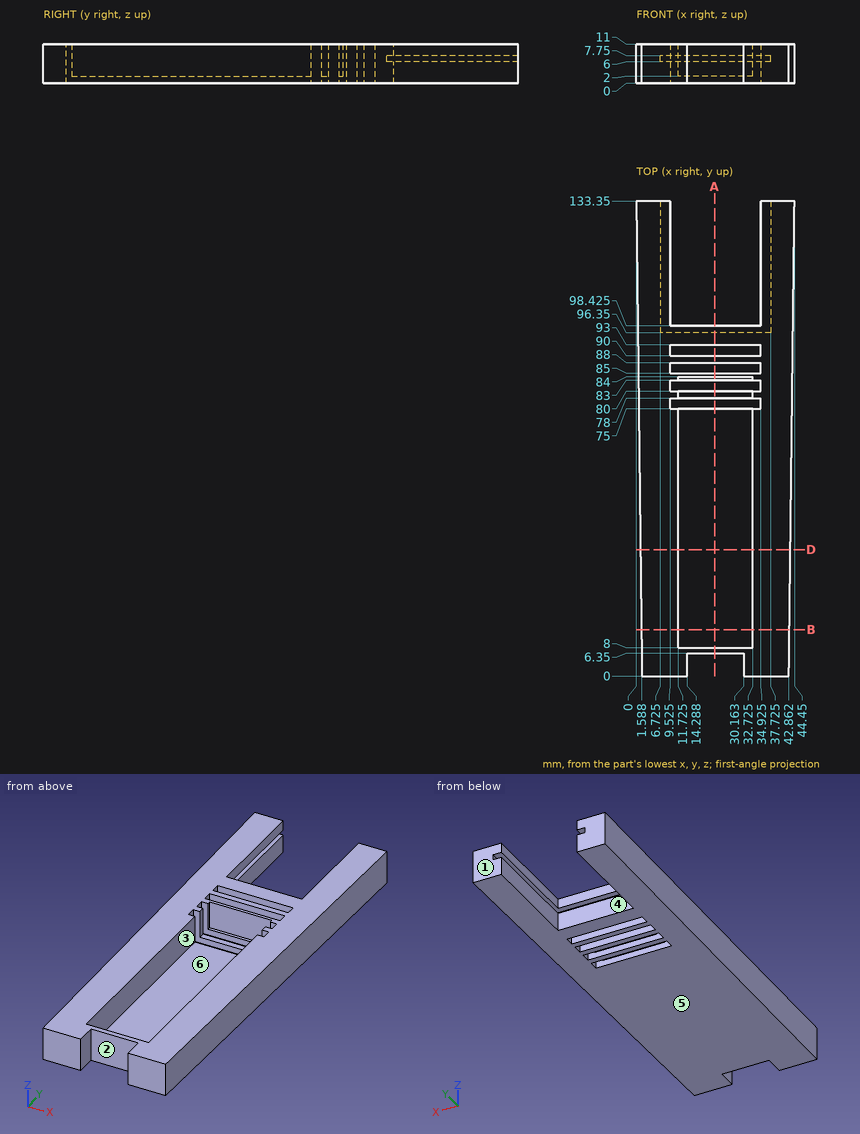
For this review, use the dimensioned drawing (mm, ordinates from the lowest corner) and the shaded views. A direction names the side the tool comes from. Give positions to 0.01 mm unless a question says otherwise; leave off trailing zeros. Order: outer loops, then holes, each group sorted by start corner. A loop starts at its lowest first (then second) coordinate and runs counter-clockwise, first axis right, second up.
1. Mouldability with a two-part tool opening along Y and no side actions: class the marked faces 1, 2 and 3 as +Y half, -Y half, draft (parallel to the pull), parting line (faces both ways), or undercut.
Solution:
face 1: +Y half
face 2: -Y half
face 3: undercut
2. For pin 1 Ø3.5 at (x, z) = (16.5, 3) entering from +Y (1 decimal); pin 2 Ø4 at (x, z) = (6.5, 3.5) entering from -Y; pin 3 Ø2 at (x, z) = (20, 2.5) entering from -Y; pin 4 Ø1 at (y, z) = (78.5, 7) entering from +X, all flat-tipped, find the tip position at first contact; note any pin that passes through.
Solution:
pin 1: stops at y = 98.4
pin 2: stops at y = 0
pin 3: stops at y = 6.35
pin 4: stops at x = 43.8
3. Tool access review of the marked faces 4, 5 and 6: name each direction out of +Z, -Z, +X, -X, +Y, -Y from which nothing blocks a thin tool from reaching the whole face with its end or side.
Solution:
face 4: +Z, -Z, +Y
face 5: -Z, +X, -X, +Y, -Y
face 6: +Z
4. To check wall thickness, follow L1, parallel to Y at x = 17, z = 7; L2, parallel to Y at x = 13, z = 4 (1 decimal); L3, parallel to Z at x = 19, y = 19. State the ranges of each line that lie inside material, in increasing order.
Solution:
L1: y = 6.35 to 8, 84 to 85, 88 to 90, 93 to 96.35
L2: y = 0 to 8, 84 to 85, 88 to 90, 93 to 98.4
L3: z = 0 to 2
5. Add section B-B, the plane y = 13. State the section outline as (x, z) points (1 decimal).
Solution:
outline: (1.4, 0) - (43, 0) - (43, 11) - (32.7, 11) - (32.7, 2) - (11.7, 2) - (11.7, 11) - (1.4, 11) - close
6. Add section D-D, the plane y = 35.5. State the section outline as (x, z) points (1 decimal), then the cut area to 3 significant figures.
Solution:
outline: (1.2, 0) - (43.3, 0) - (43.3, 11) - (32.7, 11) - (32.7, 2) - (11.7, 2) - (11.7, 11) - (1.2, 11) - close
area: 274 mm2
7. Add section A-A, the plane x = 22. State how many separate pieces and enclosed holes the cut face has, then the cut area to 3 significant figures.
Solution:
separate pieces: 5
enclosed holes: 0
area: 247 mm2
